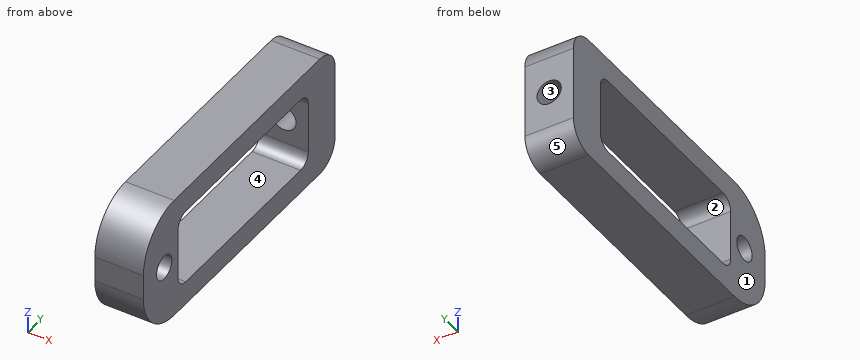
from build123d import *

# Parameters (mm, degrees)
SKETCH21_W          = 4
SKETCH21_H          = 10.1
BOSS_EXTRUDE1_DEPTH = 25
SKETCH22_R          = 1
CUT_EXTRUDE4_DEPTH  = 4
SKETCH23_W          = 6.2
SKETCH23_H          = 17
CUT_EXTRUDE5_DEPTH  = 4
SKETCH24_R          = 1
CUT_EXTRUDE6_DEPTH  = 3.5
FILLET4_R           = 4
FILLET5_R           = 2
FILLET6_R           = 1


with BuildPart() as part:
    # Sketch21 → Boss-Extrude1 (new body)
    with BuildSketch(Plane(origin=(0, 0, 0), x_dir=(1, 0, 0), z_dir=(0, 1, 0))):
        Rectangle(SKETCH21_W, SKETCH21_H)
    extrude(amount=BOSS_EXTRUDE1_DEPTH)

    # Sketch22 → Cut-Extrude4 (cut)
    with BuildSketch(Plane.ZY.offset(2)):
        with Locations((0, 2.7)):
            Circle(SKETCH22_R)
    extrude(amount=-CUT_EXTRUDE4_DEPTH, mode=Mode.SUBTRACT)

    # Sketch23 → Cut-Extrude5 (cut)
    with BuildSketch(Plane.ZY.offset(2)):
        with Locations((0, 13)):
            Rectangle(SKETCH23_W, SKETCH23_H)
    extrude(amount=-CUT_EXTRUDE5_DEPTH, mode=Mode.SUBTRACT)

    # Sketch24 → Cut-Extrude6 (cut)
    with BuildSketch(Plane(origin=(0, 25, 0), x_dir=(1, 0, 0), z_dir=(0, 1, 0))):
        with Locations(Location((0, 0, 0), (0, 0, 270))):
            Circle(SKETCH24_R)
    extrude(amount=-CUT_EXTRUDE6_DEPTH, mode=Mode.SUBTRACT)

    # Fillet4
    fillet4_edges = [part.edges().sort_by_distance(p)[0] for p in [
        (0, 0, 5.05),
        (0, 0, -5.05),
    ]]
    fillet(fillet4_edges, radius=FILLET4_R)

    # Fillet5
    fillet5_edges = [part.edges().sort_by_distance(p)[0] for p in [
        (0, 25, 5.05),
        (0, 25, -5.05),
    ]]
    fillet(fillet5_edges, radius=FILLET5_R)

    # Fillet6
    fillet6_edges = [part.edges().sort_by_distance(p)[0] for p in [
        (0, 21.5, 3.1),
        (0, 4.5, 3.1),
        (0, 4.5, -3.1),
        (0, 21.5, -3.1),
    ]]
    fillet(fillet6_edges, radius=FILLET6_R)


solid = part.part
Geometry: final body of the model. Coordinates: model frame, mm. Face numbers are marked on the shaded views. A direction names the side the tool comes from. Give positions to 0.01 mm unless a question says otherwise; leave off trailing zeros. Order: outer loops, then holes, each group sorted by start corner. A loop starts at its lowest first (then second) coordinate and runs counter-clockwise, first axis right, second up. Notation, with made-up numbers: (17.5, 41.5) -> (41.5, 41.5) arc R19 cw to (41.5, 73.5) -> close; hole circle Ø7 at (-38, 10). An arc over 180 degrees is marked (long way). Put each result on its own line as item: value.
Q1. Section B-B, the plane z = 0. Return loops of the section in (x, y).
Here are the results:
outline: (-2, 0) -> (2, 0) -> (2, 1.7) -> (-2, 1.7) -> close; (-2, 3.7) -> (2, 3.7) -> (2, 4.5) -> (-2, 4.5) -> close; (-2, 21.5) -> (-1, 21.5) -> (-1, 25) -> (-2, 25) -> close; (1, 21.5) -> (2, 21.5) -> (2, 25) -> (1, 25) -> close
Q2. Section A-A, the plane y = 10. Return loops of the section in (x, z).
Here are the results:
outline: (-2, -5.05) -> (2, -5.05) -> (2, -3.1) -> (-2, -3.1) -> close; (-2, 3.1) -> (2, 3.1) -> (2, 5.05) -> (-2, 5.05) -> close
Q3. Reachability of the marked faces 4 and 5 from +Z, -Z, +X, -X, +Y, -Y: full face, straight path, thin tool, end or side. Return the list, or none.
Here are the results:
face 4: +X, -X
face 5: -Z, +X, -X, +Y
Q4. Section D-D, the plane z = 1.75. Return loops of the section in (x, y), then the cut area to 3 significant figures.
Here are the results:
outline: (-2, 0.06) -> (2, 0.06) -> (2, 4.5) -> (-2, 4.5) -> close; (-2, 21.5) -> (2, 21.5) -> (2, 25) -> (-2, 25) -> close
area: 31.8 mm^2
Q5. Draft query along X for the marked faces 1, 2 and 3. Return one class per face: released by +X, released by -X, zero draft, split by the parting line, or undercut.
Here are the results:
face 1: released by -X
face 2: zero draft
face 3: undercut
Q6. Section C-C, the plane x = -0.6. Return loops of the section in (y, z), then the cut area to 3 significant figures.
Here are the results:
outline: (0, -1.05) arc R4 ccw to (4, -5.05) -> (23, -5.05) arc R2 ccw to (25, -3.05) -> (25, -0.8) -> (21.5, -0.8) -> (21.5, -2.1) arc R1 cw to (20.5, -3.1) -> (5.5, -3.1) arc R1 cw to (4.5, -2.1) -> (4.5, 2.1) arc R1 cw to (5.5, 3.1) -> (20.5, 3.1) arc R1 cw to (21.5, 2.1) -> (21.5, 0.8) -> (25, 0.8) -> (25, 3.05) arc R2 ccw to (23, 5.05) -> (4, 5.05) arc R4 ccw to (0, 1.05) -> close; hole circle Ø2 at (2.7, 0)
area: 131 mm^2
Q7. Material intervals for L1, parallel to Z at x = -0.8, y = 11; L2, parallel to Y at x = 0.1, z = 0; L3, parallel to X at y = 22.7, z = 0, sorted ascending.
Here are the results:
L1: z = -5.05 to -3.1, 3.1 to 5.05
L2: y = 0 to 1.7, 3.7 to 4.5
L3: x = -2 to -1, 1 to 2
